```python
from build123d import *

# Parameters (mm, degrees)
SKETCH1_R           = 11.5
SKETCH1_R_2         = 9.5
BOSS_EXTRUDE2_DEPTH = 6
SKETCH1_6_R         = 11.5
SKETCH1_6_R_2       = 1.325
BOSS_EXTRUDE3_DEPTH = 2
FILLET4_SIZE        = 4


with BuildPart() as part:
    # Sketch1 → Boss-Extrude2 (new body)
    # profile 1 of 9: a face of its own
    with BuildSketch(Plane(origin=(0, 0, 0), x_dir=(1, 0, 0), z_dir=(0, 1, 0))):
        with BuildLine():
            ThreePointArc((-11.166355717, -2.75), (-11.5, 0), (-11.166355717, 2.75))
            Line((-11.166355717, 2.75), (-22.5, 1))
            Line((-22.5, 1), (-22.5, -1))
            Line((-22.5, -1), (-11.166355717, -2.75))
        make_face()
    # profile 2 of 9: a face of its own
    with BuildSketch(Plane(origin=(0, 0, 0), x_dir=(1, 0, 0), z_dir=(0, 1, 0))):
        with BuildLine():
            Line((-15.202795796, -16.617009358), (-5.9512622, -9.840349497))
            ThreePointArc((-5.9512622, -9.840349497), (-8.131727984, -8.131727984), (-9.840349497, -5.9512622))
            Line((-9.840349497, -5.9512622), (-16.617009358, -15.202795796))
            Line((-16.617009358, -15.202795796), (-15.202795796, -16.617009358))
        make_face()
    # profile 3 of 9: a face of its own
    with BuildSketch(Plane(origin=(0, 0, 0), x_dir=(1, 0, 0), z_dir=(0, 1, 0))):
        with BuildLine():
            ThreePointArc((-9.840349497, 5.9512622), (-8.131727984, 8.131727984), (-5.9512622, 9.840349497))
            Line((-5.9512622, 9.840349497), (-15.202795796, 16.617009358))
            Line((-15.202795796, 16.617009358), (-16.617009358, 15.202795796))
            Line((-16.617009358, 15.202795796), (-9.840349497, 5.9512622))
        make_face()
    # profile 4 of 9: a face of its own
    with BuildSketch(Plane(origin=(0, 0, 0), x_dir=(1, 0, 0), z_dir=(0, 1, 0))):
        with BuildLine():
            ThreePointArc((-2.75, 11.166355717), (0, 11.5), (2.75, 11.166355717))
            Line((2.75, 11.166355717), (1, 22.5))
            Line((1, 22.5), (-1, 22.5))
            Line((-1, 22.5), (-2.75, 11.166355717))
        make_face()
    # profile 5 of 9: a face of its own
    with BuildSketch(Plane(origin=(0, 0, 0), x_dir=(1, 0, 0), z_dir=(0, 1, 0))):
        with BuildLine():
            ThreePointArc((5.9512622, 9.840349497), (8.131727984, 8.131727984), (9.840349497, 5.9512622))
            Line((9.840349497, 5.9512622), (16.617009358, 15.202795796))
            Line((16.617009358, 15.202795796), (15.202795796, 16.617009358))
            Line((15.202795796, 16.617009358), (5.9512622, 9.840349497))
        make_face()
    # profile 6 of 9: a face of its own
    with BuildSketch(Plane(origin=(0, 0, 0), x_dir=(1, 0, 0), z_dir=(0, 1, 0))):
        with BuildLine():
            Line((22.5, 1), (11.166355717, 2.75))
            ThreePointArc((11.166355717, 2.75), (11.416284219, 1.385082895), (11.5, 0))
            ThreePointArc((11.5, 0), (11.416284219, -1.385082895), (11.166355717, -2.75))
            Line((11.166355717, -2.75), (22.5, -1))
            Line((22.5, -1), (22.5, 1))
        make_face()
    # profile 7 of 9: a face of its own
    with BuildSketch(Plane(origin=(0, 0, 0), x_dir=(1, 0, 0), z_dir=(0, 1, 0))):
        with BuildLine():
            Line((1, -22.5), (2.75, -11.166355717))
            ThreePointArc((2.75, -11.166355717), (0, -11.5), (-2.75, -11.166355717))
            Line((-2.75, -11.166355717), (-1, -22.5))
            Line((-1, -22.5), (1, -22.5))
        make_face()
    # profile 8 of 9: a face of its own
    with BuildSketch(Plane(origin=(0, 0, 0), x_dir=(1, 0, 0), z_dir=(0, 1, 0))):
        with BuildLine():
            Line((16.617009358, -15.202795796), (9.840349497, -5.9512622))
            ThreePointArc((9.840349497, -5.9512622), (8.131727984, -8.131727984), (5.9512622, -9.840349497))
            Line((5.9512622, -9.840349497), (15.202795796, -16.617009358))
            Line((15.202795796, -16.617009358), (16.617009358, -15.202795796))
        make_face()
    # profile 9 of 9: a face of its own
    with BuildSketch(Plane(origin=(0, 0, 0), x_dir=(1, 0, 0), z_dir=(0, 1, 0))):
        Circle(SKETCH1_R)
        with Locations(Location((0, 0, 0), (0, 0, 270))):
            Circle(SKETCH1_R_2, mode=Mode.SUBTRACT)
    extrude(amount=BOSS_EXTRUDE2_DEPTH)

    # Sketch1<6> → Boss-Extrude3 (add)
    with BuildSketch(Plane(origin=(0, 0, 0), x_dir=(1, 0, 0), z_dir=(0, 1, 0))):
        Circle(SKETCH1_6_R)
        with Locations(Location((0, 0, 0), (0, 0, 270))):
            Circle(SKETCH1_6_R_2, mode=Mode.SUBTRACT)
    extrude(amount=BOSS_EXTRUDE3_DEPTH)

    # Fillet4
    # a fillet whose section is not a circle: 4 mm, written as the material it adds along each edge
    with BuildSketch(Plane(origin=(0, 2, 0), x_dir=(0, 0, 1), z_dir=(1, 0, 0))) as fillet4_piece_1:
        with BuildLine():
            Bezier((9.5 - FILLET4_SIZE, 0), (9.5, 0), (9.5, -FILLET4_SIZE), weights=[1, 1, 1])
            Line((9.5, -FILLET4_SIZE), (9.5, 0))
            Line((9.5, 0), (9.5 - FILLET4_SIZE, 0))
        make_face()
    revolve(axis=Axis((0, 2, 0), (0, -1, 0)))


solid = part.part
```
Here's how the part is built. I have some questions about the finished solid (model axes, mm). A direction names the side the tool comes from. Round coordinates to 2 decimals unless told otherwise and drop trailing zeros. Write each loop counter-clockwise with the first axis right and the second up, starting at its lowest first coordinate (ties: lowest second). Pieces come first, ordered by that corner, then holes.
Q1. If we section it at A-A on x = -14: Write out the boundary of the cut face in (y, z).
Q2. Which directions (+Z, -Z, +X, -X, +Y, -Y) give clear straight access to the entire face, cutting with the end or side of a thin tool? Please do faces 5 (the cylindrical face through (-4.378, 2.958, -10.634)), 6 (the cylindrical face through (-10.615, 2.958, -4.423)), 7 (the flat face through (16.754, 2.958, 1.887)), 8 (the cylindrical face through (-4.423, 2.958, 10.615)).
Q3. Please list where these lines run through material, in increasing order: probe 1 along X at (y, z) = (0.9, 0) (3 decimals); probe 2 along Z at (x, y) = (16.5, 0.75); probe 3 along X at (y, z) = (2.5, 14.5).
Q4. Will these pins go through, and if not, where does the flat tip stop? P1, Ø3, axis at x = 14.5, y = 5, coming from the +Z side; P2, Ø9, axis at x = 2, z = 2.5, coming from the +Y side; P3, Ø2.5, axis at x = 0, z = 0, coming from the +Y side; P4, Ø2, axis at y = 2.5, z = -15, coming from the +X side.
Q5. If we section it at B-B on z = 12: Write out the boundary of the cut face in (x, y).
Q6. If we mould it in two halves opening along X, with no side actions, what happens to faces 1 (the flat face through (-10.642, 2.958, 13.276)), 2 (the cylindrical face through (-10.634, 2.958, 4.378)), 3 (the flat face through (1.1, 2, 1.1)), 4 (the flat face through (5, 0, 0))? For each: +X half, -X half, draft (parallel to the pull), parting line (faces both ways), or undercut.
Answer below:
1. outline: (0, -15.74) - (6, -15.74) - (6, -11.63) - (0, -11.63) - close; (0, -2.31) - (6, -2.31) - (6, 2.31) - (0, 2.31) - close; (0, 11.63) - (6, 11.63) - (6, 15.74) - (0, 15.74) - close
2. face 5: -Z, +Y, -Y
2. face 6: -X, +Y, -Y
2. face 7: +X, +Y, -Y
2. face 8: +Z, +Y, -Y
3. probe 1: x = -22.5 to -1.325, 1.325 to 22.5
3. probe 2: z = -15.32 to -15.04, -1.93 to 1.93, 15.04 to 15.32
3. probe 3: x = -16.1 to -12.31, -2.24 to 2.24, 12.31 to 16.1
4. P1: stops at z = 16.62
4. P2: stops at y = 2.43
4. P3: passes through
4. P4: stops at x = 16.62
5. outline: (-14.27, 0) - (-8.9, 0) - (-8.9, 6) - (-14.27, 6) - close; (-2.62, 0) - (2.62, 0) - (2.62, 6) - (-2.62, 6) - close; (8.9, 0) - (14.27, 0) - (14.27, 6) - (8.9, 6) - close
6. face 1: undercut
6. face 2: -X half
6. face 3: undercut
6. face 4: draft
